```python
from build123d import *

# Parameters (mm, degrees)
SKETCH_1_W          = 210
SKETCH_1_H          = 100
EXTRUDE_1_DEPTH     = 5
CUT_EXTRUDE_1_DEPTH = 40
SKETCH_8_R          = 1.5
CUT_EXTRUDE_7_DEPTH = 5
FILLET_1_R          = 5
SKETCH_9_R          = 1.5
CUT_EXTRUDE_8_DEPTH = 233.647802483


with BuildPart() as part:
    # 草图1 → 凸台-拉伸1 (new body)
    with BuildSketch(Plane(origin=(0, 0, 0), x_dir=(1, 0, 0), z_dir=(0, 1, 0))):
        with Locations((105, -50)):
            Rectangle(SKETCH_1_W, SKETCH_1_H)
    extrude(amount=EXTRUDE_1_DEPTH)

    # 草图2 → 切除-拉伸1 (cut)
    with BuildSketch(Plane(origin=(0, 5, 0), x_dir=(1, 0, 0), z_dir=(0, 1, 0))):
        with BuildLine():
            Line((30, -40), (70, -40))
            ThreePointArc((70, -40), (80, -50), (70, -60))
            Line((70, -60), (30, -60))
            ThreePointArc((30, -60), (20, -50), (30, -40))
        make_face()
        with BuildLine():
            Line((140, -40), (180, -40))
            ThreePointArc((180, -40), (190, -50), (180, -60))
            Line((180, -60), (140, -60))
            ThreePointArc((140, -60), (130, -50), (140, -40))
        make_face()
    extrude(amount=-CUT_EXTRUDE_1_DEPTH, mode=Mode.SUBTRACT)

    # 草图8 → 切除-拉伸7 (cut)
    with BuildSketch(Plane(origin=(0, 5, 0), x_dir=(1, 0, 0), z_dir=(0, 1, 0))):
        with Locations(Location((15, -10, 0), (0, 0, 270))):
            Circle(SKETCH_8_R)
        with Locations(Location((15, -90, 0), (0, 0, 270))):
            Circle(SKETCH_8_R)
        with Locations(Location((195, -90, 0), (0, 0, 270))):
            Circle(SKETCH_8_R)
        with Locations(Location((195, -10, 0), (0, 0, 270))):
            Circle(SKETCH_8_R)
    extrude(amount=-CUT_EXTRUDE_7_DEPTH, mode=Mode.SUBTRACT)

    # 圆角1
    fillet_1_edges = [part.edges().sort_by_distance(p)[0] for p in [
        (0, 2.5, 0),
        (210, 2.5, 0),
        (210, 2.5, 100),
        (0, 2.5, 100),
    ]]
    fillet(fillet_1_edges, radius=FILLET_1_R)

    # 草图9 → 切除-拉伸8 (cut, through all)
    with BuildSketch(Plane(origin=(0, 5, 0), x_dir=(1, 0, 0), z_dir=(0, 1, 0))):
        with Locations(Location((93, -34, 0), (0, 0, 270))):
            Circle(SKETCH_9_R)
        with Locations(Location((117, -34, 0), (0, 0, 90))):
            Circle(SKETCH_9_R)
        with Locations(Location((117, -66, 0), (0, 0, 270))):
            Circle(SKETCH_9_R)
        with Locations(Location((93, -66, 0), (0, 0, 90))):
            Circle(SKETCH_9_R)
    extrude(amount=-CUT_EXTRUDE_8_DEPTH, mode=Mode.SUBTRACT)


solid = part.part
```
The model under review builds one solid part; all positions refer to its coordinate system, in mm. A direction names the side the tool comes from. Round coordinates to 2 decimals unless told otherwise and drop trailing zeros. Order: outer loops, then holes, each group sorted by start corner. A loop starts at its lowest first (then second) coordinate and runs counter-clockwise, first axis right, second up. Notation, with made-up numbers: M 27,-29 L 85,-29 A19 cw 85,-25 Z; hole C 42,55.25 d3. An arc over 180 degrees is marked long. Use a Markdown table: item, result.
1) Wall thickness on line 1 along X through (y, z) = (3.75, 10); line 2 along X through (y, z) = (2.4, 34); line 3 along Z through (x, y) = (195, 2.25): over which ranges is each line inside the solid? List them lowest first. Write a range as [from, to].
Report:
| item | result |
|---|---|
| line 1 | [0, 13.5], [16.5, 193.5], [196.5, 210] |
| line 2 | [0, 91.5], [94.5, 115.5], [118.5, 210] |
| line 3 | [0, 8.5], [11.5, 88.5], [91.5, 100] |
2) Consider section A-A (z = 50). Write out the cut boundary in (x, y), then the cut area to 3 significant figures.
Report:
| item | result |
|---|---|
| outline | M 0,0 L 20,0 L 20,5 L 0,5 Z; M 80,0 L 130,0 L 130,5 L 80,5 Z; M 190,0 L 210,0 L 210,5 L 190,5 Z |
| area | 450 mm^2 |
3) Consider section C-C (y = 2.7). Give the number of separate pieces and of enclosed holes in the cut face, then the cut area to 3 significant figures.
Report:
| item | result |
|---|---|
| separate pieces | 1 |
| enclosed holes | 10 |
| area | 18,700 mm^2 |
4) Draft analysis for pull direction Z (two halves, no side actions). For faces 1 (the face through (1, 3, 98)), 2 (the face through (104, 0, 49)), 3 (the face through (130, 3, 50)), state which applies: released by +Z, released by -Z, zero draft, split by the parting line, or undercut.
Report:
| item | result |
|---|---|
| face 1 | released by +Z |
| face 2 | zero draft |
| face 3 | undercut |
5) Consider section B-B (x = 38). Write out the cut boundary in (y, z).
Report:
| item | result |
|---|---|
| outline | M 0,0 L 5,0 L 5,40 L 0,40 Z; M 0,60 L 5,60 L 5,100 L 0,100 Z |
6) Tool access review of faces 4 (the face through (104, 2, 100)), 5 (the face through (80, 3, 50)): name each direction out of +Z, -Z, +X, -X, +Y, -Y from which nothing blocks a thin tool from reaching the whole face with its end or side.
Report:
| item | result |
|---|---|
| face 4 | +Z, +X, -X, +Y, -Y |
| face 5 | +Y, -Y |
